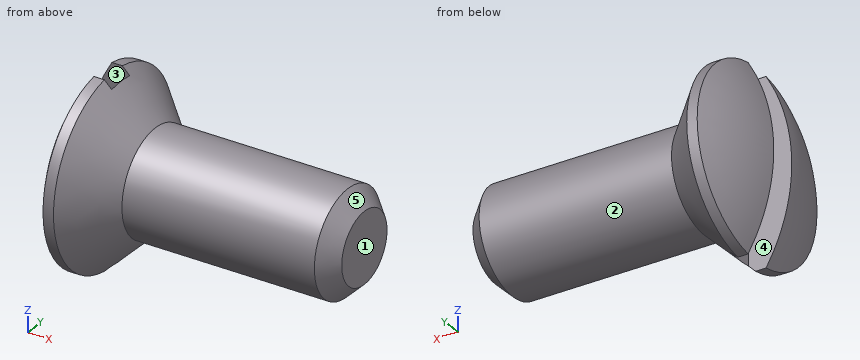
Autodesk Inventor part; units mm, degrees
ref_plane "IDS_WORKPLANE{1}" through (-2.5, 0, 0) normal (1, 0, 0) x (0, 1, 0)
ref_plane "Work Plane2" through (10.9537, 0, 0) normal (0, 0, -1) x (1, 0, 0)
ref_plane "YZ Plane" through (0, 0, 0) normal (1, 0, 0) x (0, 1, 0)
sketch "Эскиз1" plane through (0, 0, 0) normal (0, 0, 1) x (1, 0, 0)
  line L0 (25, 0) -> (25, 5)
  line L1 (25, 5) -> (6.5, 5)
  line L2 (1, 9) -> (0, 9)
  line L3 (0, 9) -> (0, 0) construction
  arc A0 (0, 9) -> (-2.5, 0) centre (14.95, 0) ccw
  line L4 (-12.7193, 0) -> (31.2866, 0)
  line L5 (0, -1.8341) -> (0, 11.0045)
  line L6 (-2.5, 0) -> (-2.5, 9) construction
  line L7 (-2.5, 9) -> (0, 9) construction
  line L8 (0, 9) -> (0, 0)
  line L9 (-2.5, 0) -> (0, 0)
  line L10 (0, 0) -> (25, 0)
  line L11 (5, 5) -> (5.5798, 5)
  line L12 (5.5798, 5) -> (6.5, 5)
  line L13 (6.5, 5) -> (-6.4328, 5) construction
  line L14 (1, 9) -> (5, 5)
  line L15 (5, 5) -> (5, 5)
  line L16 (6.5, 5) -> (5, 5) construction
  dimension "d0" = 18.5
  dimension "d1" = 25
  dimension "d2" = 2.5
  dimension "d3" = 10
  dimension "d4" = 18
  dimension "d5" = 10
  dimension "d6" = 0.9202
  dimension "d15" = 5
  dimension "d16" = 45
revolve "Базовый элемент" add sketch "Эскиз1" angle 360 about axis through (0, 0, 0) along (1, 0, 0)
ref_plane "IDS_WORKPLANE{1}" through (-2.5, 0, 0) normal (1, 0, 0) x (0, 1, 0)
sketch "Эскиз2" plane through (-2.5, 0, 0) normal (1, 0, 0) x (0, 1, 0)
  line L0 (0, -12.6) -> (0, 12.6)
  line L1 (-12.6, 0) -> (12.6, 0)
  line L2 (1.35, -9) -> (-1.35, -9)
  line L3 (-1.35, -9) -> (-1.35, 9)
  line L4 (-1.35, 9) -> (1.35, 9)
  line L5 (1.35, 9) -> (1.35, -9)
  line L6 (0, 9) -> (0, -9) construction
  line L7 (-1.35, 0) -> (1.35, 0) construction
  circle A0 centre (0, 0) radius 9
  dimension "d12" = 2.7
extrude "Паз" cut sketch "Эскиз2" along normal blind 4.2 contours A0 L3 L1 L0 | A0 L5 L2 | L2 L3 A0 | L0 L1 L5 A0 | L1 L3 A0 L0 | L0 A0 L5 L1 | A0 L3 L4 | L4 L5 A0
thread "Резьба"
chamfer "Фаска1" distance 1.6 angle 45 1 edges at (25, -5, 0)
ref_plane "Work Plane2" through (10.9537, 0, 0) normal (0, 0, -1) x (1, 0, 0)
equation "\"d0\" = GEL"
equation "\"d5\" = BDM"
equation "\"d6\" = GAL"
equation "\"NLG\" = 25"
equation "\"GEL\" = 18.5"
equation "\"KOD\" = 18"
equation "\"KOH\" = 5"
equation "\"STI\" = 4.9"
equation "\"SBR\" = 1.35"
equation "\"KAH\" = 2.5"
equation "\"GAL\" = 0.61345 * PTC"
equation "\"GUL\" = 0.61345 * PTC"
equation "\"BDM\" = NND"
equation "\"SPD\" = NND - 1.2269 * PTC"
equation "\"SEWI\" = 90deg"
equation "\"d11\" = -KAH"
equation "\"KR\" = 19"
equation "\"PTC\" = 1.5"
equation "\"TOA\" = 30deg"
equation "\"RR\" = 0.1 * NND"
equation "\"GD1\" = THREADDIA - 1.2269 * PTC"
equation "\"FAWI\" = 45deg"
properties part number "Винт M10-6gx25 ГОСТ 17474-80" material "Сталь, мягкая"
Model file for the job. Use its own axes, mm. Face numbers are marked on the shaded views. A direction names the side the tool comes from. Give positions to 0.01 mm unless a question says otherwise; leave off trailing zeros. Write each loop counter-clockwise with the first axis right and the second up, starting at its lowest first coordinate (ties: lowest second). Pieces come first, ordered by that corner, then holes. Notation, with made-up numbers: (37, -5) - (52, -5) arc R16 ccw to (52, 9) - close; hole circle Ø7 at (79.5, -26). An arc over 180 degrees is marked (long way). One line per question, with ' | ' between items. Start each with the question number.
(1) Slice it at D-D on x = 3. Write the cut outline in (y, z).
(2) Pin check, flat tips, straight feed: P1, Ø3, axis at y = -0.5, z = 2, coming from the -X side; P2, Ø8, axis at x = 0.5, z = -1.5, coming from the +Y side; P3, Ø10, axis at y = 6.5, z = -6.5, coming from the -X side; P4, Ø8, axis at x = 7.5, y = 1.5, coming from the -Z side. Stop position of each tip, or through.
(3) Slice it at A-A on y = 0. Write the cut outline in (x, z), plus the area to 3 significant figures.
(4) 3-axis set-ups, long thin cutter, end or side, ignore diameter. For the marked faces 4 and 5: which of +Z, -Z, +X, -X, +Y, -Y reach the whole face in a straight line?
(5) Wall check: line 1 along Y through (x, z) = (10.75, -4); line 2 along X through (y, z) = (-6, -5); line 3 along Y through (x, z) = (7.75, -1.5). Give the ranges that are in metal, low to high. Write a range as from..to.
(6) Slice it at B-B on z = 0. Write the cut outline in (x, y), plus the area to 3 significant figures.
(7) Two-plate mould, pull along Y, no slides. Class the marked faces 1, 2 and 3: +Y half, -Y half, draft (parallel to the pull), parting line (faces both ways), or undercut.
(8) Slice it at C-C on x = 22.5. Write the cut outline in (y, z).
Results below:
1) outline: circle Ø14 at (0, 0)
2) P1: x = -2.43 | P2: y = 9 | P3: x = -1.99 | P4: z = -6.39
3) outline: (1.7, -8.3) - (5, -5) - (23.4, -5) - (25, -3.4) - (25, 3.4) - (23.4, 5) - (5, 5) - (1.7, 8.3) - close | area: 241 mm^2
4) face 4: +Z, -Z, -X | face 5: +X
5) line 1: -3..3 | line 2: -0.65..2.19 | line 3: -4.77..4.77
6) outline: (-2.45, -1.35) arc R17.45 ccw to (0, -9) - (1, -9) - (5, -5) - (23.4, -5) - (25, -3.4) - (25, 3.4) - (23.4, 5) - (5, 5) - (1, 9) - (0, 9) arc R17.45 ccw to (-2.45, 1.35) - (1.7, 1.35) - (1.7, -1.35) - close | area: 291 mm^2
7) face 1: draft | face 2: parting line | face 3: undercut
8) outline: circle Ø10 at (0, 0)
